Model file for the job. Use its own axes, mm. Face numbers are marked on the shaded views. Give positions to 0.01 mm unless a question says otherwise; leave off trailing zeros. Write each loop counter-clockwise with the first axis right and the second up, starting at its lowest first coordinate (ties: lowest second). Pieces come first, ordered by that corner, then holes. Notation, with made-up numbers: M -1.75,41 L 42.25,41 A29 cw 42.25,72 Z; hole C 82,21 d11. An arc over 180 degrees is marked long. Answer as a JSON object with one key per item and string values. Group by question number.
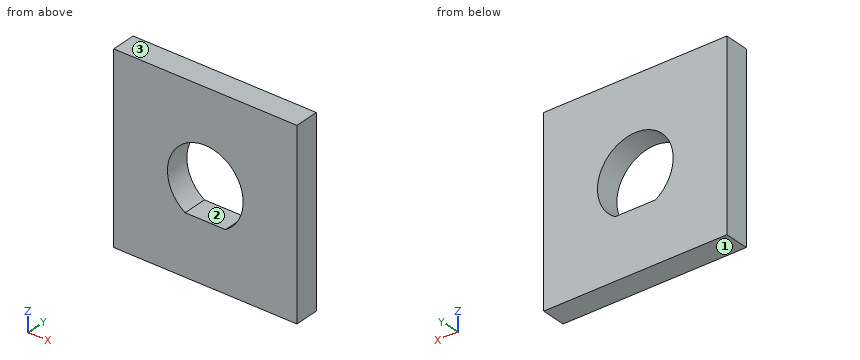
```python
from build123d import *

# Parameters (mm, degrees)
SKETCH1_W           = 15
SKETCH1_H           = 15
BOSS_EXTRUDE1_DEPTH = 2


with BuildPart() as part:
    # Sketch1 → Boss-Extrude1 (new body)
    with BuildSketch(Plane(origin=(0, 0, 0), x_dir=(1, 0, 0), z_dir=(0, 1, 0))):
        Rectangle(SKETCH1_W, SKETCH1_H)
        with BuildLine():
            Line((-1.655, 2.621254471), (1.655, 2.621254471))
            ThreePointArc((1.655, 2.621254471), (0, -3.1), (-1.655, 2.621254471))
        make_face(mode=Mode.SUBTRACT)
    extrude(amount=BOSS_EXTRUDE1_DEPTH)


solid = part.part
```
Q1. Drop a flat-ended pin along its axis: P1, Ø2, axis at x = 0, z = 0.5, coming from the +Y side. Give the stop position or say it passes through.
Q2. Slice it at C-C, the plane y = 1.2. Write the cut outline in (x, z) (3 decimals).
Q3. Slice it at A-A, the plane x = 0. Write the cut outline in (y, z), then the cut area to 3 significant figures.
Q4. Slice it at B-B, the plane z = 0. Write the cut outline in (x, y).
Q5. Two-plate mould, pull along Z, no slides. Class the marked faces 1, 2 and 3: +Z half, -Z half, draft (parallel to the pull), parting line (faces both ways), or undercut.
Q6. Wall check: L1, parallel to Z at x = 0, y = 1.45; L2, parallel to X at y = 1.4, z = 0; L3, parallel to X at y = 1.6, z = 1.5. Give the ranges that are in metal, low to high.
Solved:
{
 "1": {"P1": "passes through"},
 "2": {"outline": "M -7.5,-7.5 L 7.5,-7.5 L 7.5,7.5 L -7.5,7.5 Z; hole M -1.655,-2.621 L 1.655,-2.621 A3.1 ccw long Z"},
 "3": {"outline": "M 0,-7.5 L 2,-7.5 L 2,-2.62 L 0,-2.62 Z; M 0,3.1 L 2,3.1 L 2,7.5 L 0,7.5 Z", "area": "18.6 mm²"},
 "4": {"outline": "M -7.5,0 L -3.1,0 L -3.1,2 L -7.5,2 Z; M 3.1,0 L 7.5,0 L 7.5,2 L 3.1,2 Z"},
 "5": {"face 1": "-Z half", "face 2": "undercut", "face 3": "+Z half"},
 "6": {"L1": "z = -7.5 to -2.62, 3.1 to 7.5", "L2": "x = -7.5 to -3.1, 3.1 to 7.5", "L3": "x = -7.5 to -2.71, 2.71 to 7.5"}
}
